Autodesk Fusion 360 part; units mm, degrees
sketch "main-bottom" plane through (0, 0, 0) normal (0, 0, 1) x (1, 0, 0)
  line L0 (30, -29) -> (-30, -29)
  line L1 (-34, -25) -> (-34, 25)
  line L2 (-30, 29) -> (30, 29)
  line L3 (34, 25) -> (34, -25)
  arc A0 (-30, 29) -> (-34, 25) centre (-30, 25) ccw
  arc A1 (-34, -25) -> (-30, -29) centre (-30, -25) ccw
  arc A2 (30, -29) -> (34, -25) centre (30, -25) ccw
  arc A3 (34, 25) -> (30, 29) centre (30, 25) ccw
  circle A4 centre (-29.5, 24.5) radius 2.3
  circle A5 centre (29.5, 24.5) radius 2.3
  circle A6 centre (29.5, -24.5) radius 2.3
  circle A7 centre (-29.5, -24.5) radius 2.3
  line L4 (-32.5, -25) -> (-32.5, 25)
  line L5 (32.5, 25) -> (32.5, -25)
  arc A8 (-30, 27.5) -> (-32.5, 25) centre (-30, 25) ccw
  arc A9 (-32.5, -25) -> (-30, -27.5) centre (-30, -25) ccw
  arc A10 (30, -27.5) -> (32.5, -25) centre (30, -25) ccw
  arc A11 (32.5, 25) -> (30, 27.5) centre (30, 25) ccw
  arc A12 (-29.5, 20) -> (-25, 24.5) centre (-29.5, 24.5) ccw
  line L6 (-25, 24.5) -> (-25, 27.5)
  line L7 (-29.5, 20) -> (-32.5, 20)
  line L8 (-29.5, 20) -> (-32.5, 20)
  arc A13 (-29.5, 20) -> (-25, 24.5) centre (-29.5, 24.5) ccw
  line L9 (-25, 24.5) -> (-25, 27.5)
  arc A14 (-29.5, 20) -> (-25, 24.5) centre (-29.5, 24.5) ccw
  line L10 (-25, 24.5) -> (-25, 27.5)
  line L11 (-29.5, 20) -> (-32.5, 20)
  arc A15 (-25, -24.5) -> (-29.5, -20) centre (-29.5, -24.5) ccw
  line L12 (-29.5, -20) -> (-32.5, -20)
  line L13 (-25, -24.5) -> (-25, -27.5)
  arc A16 (29.5, -20) -> (25, -24.5) centre (29.5, -24.5) ccw
  line L14 (25, -24.5) -> (25, -27.5)
  line L15 (29.5, -20) -> (32.5, -20)
  arc A17 (25, 24.5) -> (29.5, 20) centre (29.5, 24.5) ccw
  line L16 (29.5, 20) -> (32.5, 20)
  line L17 (25, 24.5) -> (25, 27.5)
  line L18 (0, -27.5) -> (0.5, -27.5) construction
  line L19 (0, 27.5) -> (0.5, 27.5) construction
  line L20 (0, -27.5) -> (0.5, -27.5)
  line L21 (0, -27.5) -> (0.5, -27.5) construction
  line L22 (3.5, -27.5) -> (3.5, 27.5)
  line L23 (0.5, 27.5) -> (0.5, -27.5)
  line L24 (30, -27.5) -> (3.5, -27.5)
  line L25 (0.5, -27.5) -> (-30, -27.5)
  line L26 (-30, 27.5) -> (0.5, 27.5)
  line L27 (3.5, 27.5) -> (30, 27.5)
  arc A18 (-29.5, 30.5) -> (-35.5, 24.5) centre (-29.5, 24.5) ccw
  line L28 (-29.5, 24.5) -> (-35.5, 24.5) construction
  arc A19 (-29.5, 30.5) -> (-35.5, 24.5) centre (-29.5, 24.5) ccw
  arc A20 (35.5, 24.5) -> (29.5, 30.5) centre (29.5, 24.5) ccw
  arc A21 (-35.5, -24.5) -> (-29.5, -30.5) centre (-29.5, -24.5) ccw
  arc A22 (29.5, -30.5) -> (35.5, -24.5) centre (29.5, -24.5) ccw
  line L29 (-29.5, 30.5) -> (29.5, 30.5)
  line L30 (35.5, 24.5) -> (35.5, -24.5)
  line L31 (29.5, -30.5) -> (-29.5, -30.5)
  line L32 (-35.5, 24.5) -> (-35.5, -24.5)
  dimension "d32" = 4.6
  dimension "d33" = 4.6
  dimension "d34" = 4.6
  dimension "d35" = 4.6
  dimension "d39" = 4.5
  dimension "d40" = 4.5
  dimension "d41" = 4.5
  dimension "d42" = 4.5
  dimension "d43" = 4.5
  dimension "d44" = 4.5
extrude "Extrude4" add sketch "main-bottom" along normal blind 15.5 contours L0 L1 L2 L3 A0 A1 A2 A3 | A4 | A5 | A6 | A7 | L4 A9 A15 L12 L13 L25 | L4 A8 A12 L6 L7 L8 A13 L9 A14 L10 L11 L26 | L5 A11 A17 L16 L17 L27 | L5 A10 A16 L14 L15 L24 makes body 1
extrude "Extrude3" add sketch "main-bottom" along normal blind 1.5 separate body contours L0 L1 L2 L3 A0 A1 A2 A3 | A4 | A5 | A6 | A7 | L4 A9 A15 L12 L13 L25 | L4 A12 L6 L7 L8 A13 L9 A14 L10 L11 A15 L12 L13 L20 L23 L25 L26 | L4 A8 A12 L6 L7 L8 A13 L9 A14 L10 L11 L26 | L5 A11 A17 L16 L17 L27 | L5 A16 L14 L15 A17 L16 L17 L22 L24 L27 | L5 A10 A16 L14 L15 L24 | A18 A19 A20 A21 A22 L29 L30 L31 L32 makes body 2
extrude "Extrude5" cut sketch "main-bottom" along normal blind 19.6 contours A18 A19 A20 A21 A22 L29 L30 L31 L32 bodies 2
extrude "Extrude6" add sketch "main-bottom" along normal blind 19.6 contours A18 A19 A20 A21 A22 L29 L30 L31 L32 bodies 1 2
hole "Hole1" at (29.5, 24.5, 15.5) direction (0, 0, -1) diameter 4.6 depth 6.5 tip angle 180 countersink diameter 5.6 countersink angle 90 bodies 1
hole "Hole2" at (-29.5, 24.5, 15.5) direction (0, 0, -1) diameter 4.6 depth 6 tip angle 180 countersink diameter 5.6 countersink angle 90 bodies 1
hole "Hole3" at (-29.5, -24.5, 15.5) direction (0, 0, -1) diameter 4.6 depth 6 tip angle 180 countersink diameter 5.6 countersink angle 90 bodies 1
hole "Hole4" at (29.5, -24.5, 15.5) direction (0, 0, -1) diameter 4.6 depth 6 tip angle 180 countersink diameter 5.6 countersink angle 90 bodies 1
sketch "Sketch2" plane through (-35.5, 0, 0) normal (-1, 0, 0) x (0, 0, 1)
  line L0 (0, 24.5) -> (0, -24.5)
  line L1 (0, -24.5) -> (19.6, -24.5)
  line L2 (19.6, -24.5) -> (19.6, 24.5)
  line L3 (19.6, 24.5) -> (0, 24.5)
  line L4 (15.5049, -24.5) -> (15.5049, -19.5) construction
  line L5 (14.1299, -19.5) -> (13.6299, -19.5)
  line L6 (12.2549, -18.125) -> (12.2549, -11.625)
  line L7 (13.6299, -10.25) -> (14.1299, -10.25)
  line L8 (15.5049, -11.625) -> (15.5049, -18.125)
  line L9 (12.2549, -10.25) -> (15.5049, -19.5) construction
  line L10 (12.2549, -19.5) -> (15.5049, -10.25) construction
  line L11 (15.5049, -19.5) -> (14.1299, -19.5) construction
  line L12 (14.1299, -19.5) -> (14.1299, -18.125) construction
  line L13 (14.1299, -18.125) -> (15.5049, -18.125) construction
  line L14 (15.5049, -18.125) -> (15.5049, -19.5) construction
  line L15 (12.2549, -19.5) -> (13.6299, -19.5) construction
  line L16 (13.6299, -19.5) -> (13.6299, -18.125) construction
  line L17 (13.6299, -18.125) -> (12.2549, -18.125) construction
  line L18 (12.2549, -18.125) -> (12.2549, -19.5) construction
  arc A0 (12.2549, -18.125) -> (13.6299, -19.5) centre (13.6299, -18.125) ccw
  arc A1 (15.0049, -18.125) -> (15.004, -18.0743) centre (13.6299, -18.125) ccw
  arc A2 (12.7558, -18.0743) -> (12.7549, -18.125) centre (14.1299, -18.125) ccw
  arc A3 (14.1299, -19.5) -> (15.5049, -18.125) centre (14.1299, -18.125) ccw
  line L19 (15.5049, -10.25) -> (14.1299, -10.25) construction
  line L20 (14.1299, -10.25) -> (14.1299, -11.625) construction
  line L21 (14.1299, -11.625) -> (15.5049, -11.625) construction
  line L22 (15.5049, -11.625) -> (15.5049, -10.25) construction
  line L23 (12.2549, -10.25) -> (13.6299, -10.25) construction
  line L24 (13.6299, -10.25) -> (13.6299, -11.625) construction
  line L25 (13.6299, -11.625) -> (12.2549, -11.625) construction
  line L26 (12.2549, -11.625) -> (12.2549, -10.25) construction
  arc A4 (15.5049, -11.625) -> (14.1299, -10.25) centre (14.1299, -11.625) ccw
  arc A5 (12.7549, -11.625) -> (12.7558, -11.6757) centre (14.1299, -11.625) ccw
  arc A6 (15.004, -11.6757) -> (15.0049, -11.625) centre (13.6299, -11.625) ccw
  arc A7 (13.6299, -10.25) -> (12.2549, -11.625) centre (13.6299, -11.625) ccw
  dimension "d88" = 5
  dimension "d89" = 3.25
  dimension "d90" = 9.25
  dimension "d93" = 1.375
  dimension "d94" = 1.375
  dimension "d95" = 1.375
  dimension "d96" = 1.375
  dimension "d97" = 1.375
  dimension "d98" = 1.375
  dimension "d99" = 1.375
  dimension "d100" = 1.375
extrude "Extrude7" cut sketch "Sketch2" against normal blind 3 contours L5 L6 L7 L8 A0 A3 A4 A7 bodies 1
fillet "Fillet1" radius 1 8 edges at (-35.5, -10.25, 13.8799) (-35.5, -10.6527, 15.1022) (-35.5, -14.875, 15.5049) (-35.5, -19.0973, 15.1022) (-35.5, -19.5, 13.8799) (-35.5, -19.0973, 12.6576) (-35.5, -14.875, 12.2549) (-35.5, -10.6527, 12.6576) on bodies 1
fillet "Fillet2" radius 1 8 edges at (33.7426, 28.7426, 0) (0, 30.5, 0) (-33.7426, 28.7426, 0) (-35.5, 0, 0) (-33.7426, -28.7426, 0) (0, -30.5, 0) (33.7426, -28.7426, 0) (35.5, 0, 0) on bodies 1
equation "M3_thread_insert_diameter = 4.6 mm"
equation "d32 = M3_thread_insert_diameter"
equation "d33 = M3_thread_insert_diameter"
equation "d34 = M3_thread_insert_diameter"
equation "d35 = M3_thread_insert_diameter"
equation "bottom_thickness = 1.5 mm"
equation "batholder_height = 13 mm"
equation "batholder_bottom_gap = 1 mm"
equation "FR4_thickness = 1.6 mm"
equation "gasket_thickness = 2.5 mm"
equation "d59 = bottom_thickness"
equation "d61 = bottom_thickness + batholder_bottom_gap + batholder_height"
equation "M3_thread_insert_height = 6 mm"
equation "d68 = M3_thread_insert_height + 0.5 mm"
equation "d69 = M3_thread_insert_diameter"
equation "d71 = M3_thread_insert_diameter + 1 mm"
equation "d73 = M3_thread_insert_height"
equation "d74 = M3_thread_insert_diameter"
equation "d76 = M3_thread_insert_diameter + 1 mm"
equation "d78 = M3_thread_insert_height"
equation "d79 = M3_thread_insert_diameter"
equation "d81 = M3_thread_insert_diameter + 1 mm"
equation "d83 = M3_thread_insert_height"
equation "d84 = M3_thread_insert_diameter"
equation "d86 = M3_thread_insert_diameter + 1 mm"
Geometry check sheet. Reference: the model listing, model coordinates, mm. A direction names the side the tool comes from. Give positions to 0.01 mm unless a question says otherwise; leave off trailing zeros. Write each loop counter-clockwise with the first axis right and the second up, starting at its lowest first coordinate (ties: lowest second). Pieces come first, ordered by that corner, then holes.
1) Thickness scan on line 1 (Y direction, x = -29.5, z = 11.7); line 2 (X direction, y = 9.5, z = 4.25); line 3 (Y direction, x = -5, z = 3.25). Record the ranges inside material, lowest first.
Values follow:
line 1: y = -30.5 to -26.8, -22.2 to -20, 20 to 22.2, 26.8 to 30.5
line 2: x = -35.5 to -32.5, 0.5 to 3.5, 32.5 to 35.5
line 3: y = -30.5 to -27.5, 27.5 to 30.5
2) Cross-section at A-A (y = -12.5). Record the boundary of the cut face in (x, z).
Values follow:
outline: (-35.5, 1) arc R1 ccw to (-34.5, 0) - (34.5, 0) arc R1 ccw to (35.5, 1) - (35.5, 19.6) - (34, 19.6) - (34, 15.5) - (32.5, 15.5) - (32.5, 1.5) - (3.5, 1.5) - (3.5, 15.5) - (0.5, 15.5) - (0.5, 1.5) - (-32.5, 1.5) - (-32.5, 12.25) - (-34.5, 12.25) arc R1 ccw to (-35.5, 11.25) - close; (-35.5, 16.5) arc R1 ccw to (-34.5, 15.5) - (-34, 15.5) - (-34, 19.6) - (-35.5, 19.6) - close
3) Cross-section at D-D (y = -6). Record the boundary of the cut face in (x, z).
Values follow:
outline: (-35.5, 1) arc R1 ccw to (-34.5, 0) - (34.5, 0) arc R1 ccw to (35.5, 1) - (35.5, 19.6) - (34, 19.6) - (34, 15.5) - (32.5, 15.5) - (32.5, 1.5) - (3.5, 1.5) - (3.5, 15.5) - (0.5, 15.5) - (0.5, 1.5) - (-32.5, 1.5) - (-32.5, 15.5) - (-34, 15.5) - (-34, 19.6) - (-35.5, 19.6) - close
4) Go/stop test with flat-tipped pins: pin 1 Ø1.5 at (y, z) = (-26.5, 6) entering from -X; pin 2 Ø2.5 at (y, z) = (26, 8.5) entering from +X; pin 3 Ø1 at (x, y) = (-33, -15) entering from +Z. Record where each tip stops, or that it passes through.
Values follow:
pin 1: stops at x = -35.37
pin 2: stops at x = 35.49
pin 3: stops at z = 12.25
5) Cross-section at C-C (x = -22.5). Record the boundary of the cut face in (y, z).
Values follow:
outline: (-30.5, 1) arc R1 ccw to (-29.5, 0) - (29.5, 0) arc R1 ccw to (30.5, 1) - (30.5, 19.6) - (29, 19.6) - (29, 15.5) - (27.5, 15.5) - (27.5, 1.5) - (-27.5, 1.5) - (-27.5, 15.5) - (-29, 15.5) - (-29, 19.6) - (-30.5, 19.6) - close
6) Cross-section at B-B (z = 17.5). Record the boundary of the cut face in (x, y).
Values follow:
outline: (-35.5, -24.5) arc R6 ccw to (-29.5, -30.5) - (29.5, -30.5) arc R6 ccw to (35.5, -24.5) - (35.5, 24.5) arc R6 ccw to (29.5, 30.5) - (-29.5, 30.5) arc R6 ccw to (-35.5, 24.5) - close; hole (-34, -25) arc R4 ccw to (-30, -29) - (30, -29) arc R4 ccw to (34, -25) - (34, 25) arc R4 ccw to (30, 29) - (-30, 29) arc R4 ccw to (-34, 25) - close
7) Set-up check for faces 1 (the face through (-16, 0, 1.5)), 2 (the face through (-34, -15, 12.255)), 3 (the face through (33.696, 28.789, 10.17)): record each of +Z, -Z, +X, -X, +Y, -Y from which the full face is reachable in a straight line by a thin tool's end or side.
Values follow:
face 1: +Z
face 2: -X
face 3: +Z, -Z, +X, +Y
8) Release check for a two-part mould opening along Y. For faces 4 (the face through (-32.5, 0, 8)), 5 (the face through (0, -30.5, 10)), 6 (the face through (32.5, 0, 8)), 7 (the face through (0, 30.5, 10)) record: released by +Y, released by -Y, zero draft, split by the parting line, or undercut.
Values follow:
face 4: undercut
face 5: released by -Y
face 6: undercut
face 7: released by +Y
